Geometry: final body of the model. Coordinates: model frame, mm. Give positions to 0.01 mm unless a question says otherwise; leave off trailing zeros. Loops run counter-clockwise (first coordinate to the right, second up) from the corner with the lowest first, then second, coordinate; pieces in that order, holes last.
from build123d import *

# Parameters (mm, degrees)
SKETCH1_R                  = 4
BOSS_EXTRUDE1_DEPTH        = 3.175
M3_CLEARANCE_HOLE1_D       = 3.2
F_12_0_12_DIAMETER_HOLE1_D = 12
F_6_CLEARANCE_HOLE2_D      = 3.6576
F_6_CLEARANCE_HOLE1_D      = 3.6576


with BuildPart() as part:
    # Sketch1 → Boss-Extrude1 (new body)
    with BuildSketch(Plane.XY):
        Polygon((16, -16), (-80.487803669, -16), (-80.487803669, 46.5), (-72.487803669, 54.5), (-28.507138544, 54.5), (16, 28.803791581), align=None)
        Circle(SKETCH1_R, mode=Mode.SUBTRACT)
    extrude(amount=-BOSS_EXTRUDE1_DEPTH)

    # M3 Clearance Hole1 (through all)
    with Locations(Plane.XY):
        with Locations((-69.237803669, 48.923393759), (-53.737803669, 48.923393759), (-45.987803669, 35.5), (-53.737803669, 22.076606241), (-69.237803669, 22.076606241), (-76.987803669, 35.5)):
            Hole(M3_CLEARANCE_HOLE1_D / 2)

    # Ø12.0 (12) Diameter Hole1 (through all)
    with Locations(Plane.XY):
        with Locations((-55.425625842, 32)):
            Hole(F_12_0_12_DIAMETER_HOLE1_D / 2)

    # #6 Clearance Hole2 (through all)
    with Locations(Plane.XY):
        with Locations((-72, 0), (-32, -8), (-64, -8)):
            Hole(F_6_CLEARANCE_HOLE2_D / 2)

    # #6 Clearance Hole1 (through all)
    with Locations(Plane.XY):
        with Locations((-32, 8), (-24, 0), (-64, 8), (-56, 0), (-40, 0), (8, 8), (8, -8)):
            Hole(F_6_CLEARANCE_HOLE1_D / 2)


solid = part.part
Item 1: Pin query (flat end, axial travel): pin 1 (1.5 mm diameter, centred on y = 32.5, z = -1.5, fed in from +X). Return the tip coordinate at first contact, or that it passes through.
Values follow:
pin 1: stops at x = 10.9
Item 2: Draft query along Y for faces 1 (the face through (-6.565, 41.832, -1.565)), 2 (the face through (16, 7, -2)), 3 (the face through (-75.39, 35.57, -1.61)). Return one class per face: +Y half, -Y half, draft (parallel to the pull), parting line (faces both ways), or undercut.
Values follow:
face 1: +Y half
face 2: draft
face 3: undercut
Item 3: Ray query, probe 1 along Y at (x, z) = (-64, -1.7); probe 2 along Y at (x, z) = (-72, -0.65); probe 3 along X at (y, z) = (9, -1.7). Return the intervals inside material, ascending.
Values follow:
probe 1: y = -16 to -9.83, -6.17 to 6.17, 9.83 to 54.5
probe 2: y = -16 to -1.83, 1.83 to 54.5
probe 3: x = -80.49 to -65.53, -62.47 to -33.53, -30.47 to 6.47, 9.53 to 16
Item 4: Section query A-A on x = -32. Return loops of the section in (y, z) (3 decimals), plus the area to 3 significant figures.
Values follow:
outline: (-16, -3.175) - (-9.829, -3.175) - (-9.829, 0) - (-16, 0) - close; (-6.171, -3.175) - (6.171, -3.175) - (6.171, 0) - (-6.171, 0) - close; (9.829, -3.175) - (54.5, -3.175) - (54.5, 0) - (9.829, 0) - close
area: 201 mm2
Item 5: Section query C-C on x = 0. Return loops of the section in (y, z) (3 decimals).
Values follow:
outline: (-16, -3.175) - (-4, -3.175) - (-4, 0) - (-16, 0) - close; (4, -3.175) - (38.041, -3.175) - (38.041, 0) - (4, 0) - close
Item 6: Section query D-D on z = -2.5. Give the number of separate pieces and of enclosed holes in the cut face, plus the area to 3 significant figures.
Values follow:
separate pieces: 1
enclosed holes: 18
area: 5,880 mm2
Item 7: Section query B-B on y = -8. Return loops of the section in (x, z) (3 decimals), plus the area to 3 significant figures.
Values follow:
outline: (-80.488, -3.175) - (-65.829, -3.175) - (-65.829, 0) - (-80.488, 0) - close; (-62.171, -3.175) - (-33.829, -3.175) - (-33.829, 0) - (-62.171, 0) - close; (-30.171, -3.175) - (6.171, -3.175) - (6.171, 0) - (-30.171, 0) - close; (9.829, -3.175) - (16, -3.175) - (16, 0) - (9.829, 0) - close
area: 272 mm2
